```python
from build123d import *

# Parameters (mm, degrees)
ESQUISSE1_R             = 3
ESQUISSE1_R_2           = 2.5
BOSS_EXTRU_1_DEPTH      = 10
ESQUISSE4_W             = 8
ESQUISSE4_H             = 2
BOSS_EXTRU_2_DEPTH      = 8
CONG_1_R                = 3
ESQUISSE6_R             = 2
ENL_V_MAT_EXTRU_2_DEPTH = 12
BOSS_EXTRU_3_DEPTH      = 0.01
BOSS_EXTRU_3_DEPTH_BACK = 0.01
ESQUISSE7_R             = 2
ESQUISSE7_R_2           = 1.94261234


with BuildPart() as part:
    # Esquisse1 → Boss.-Extru.1 (new body)
    with BuildSketch(Plane.XY):
        Circle(ESQUISSE1_R)
        Circle(ESQUISSE1_R_2, mode=Mode.SUBTRACT)
    extrude(amount=BOSS_EXTRU_1_DEPTH)

    # Esquisse3 for Lissage3 → Lissage3 section 0
    with BuildSketch(Plane(origin=(0, 0, 0), x_dir=(-1, 0, 0), z_dir=(0, 0, -1))):
        with BuildLine():
            # circular arc as an exact rational Bezier (weights 1, cos(half-angle), 1)
            Bezier((-2.9104275, 0.727606875), (0, 12.369316884), (2.9104275, 0.727606875), weights=[1, 0.242535625, 1])
            Bezier((2.9104275, 0.727606875), (3.09232922, 0), (2.9104275, -0.727606875), weights=[1, 0.9701425, 1])
            Bezier((2.9104275, -0.727606875), (0, -12.369316884), (-2.9104275, -0.727606875), weights=[1, 0.242535625, 1])
            Bezier((-2.9104275, -0.727606875), (-3.09232922, 0), (-2.9104275, 0.727606875), weights=[1, 0.9701425, 1])
        make_face()
    # Esquisse2 → Lissage3 section 1
    with BuildSketch(Plane.XY.offset(-8)):
        with BuildLine():
            Line((4, 1), (-4, 1))
            Line((-4, 1), (-4, -1))
            Line((-4, -1), (4, -1))
            Line((4, -1), (4, 1))
        make_face()
    loft()

    # Esquisse4 → Boss.-Extru.2 (add)
    with BuildSketch(Plane(origin=(0, 0, -8), x_dir=(-1, 0, 0), z_dir=(0, 0, -1))):
        Rectangle(ESQUISSE4_W, ESQUISSE4_H)
    extrude(amount=BOSS_EXTRU_2_DEPTH)

    # Congé1
    cong_1_edges = [part.edges().sort_by_distance(p)[0] for p in [
        (-4, 0, -16),
        (4, 0, -16),
    ]]
    fillet(cong_1_edges, radius=CONG_1_R)

    # Esquisse6 → Enlèv. mat.-Extru.2 (cut)
    with BuildSketch(Plane(origin=(0, 1, 0), x_dir=(1, 0, 0), z_dir=(0, 1, 0))):
        with Locations(Location((0, 12, 0), (0, 0, 180))):
            Circle(ESQUISSE6_R)
    extrude(amount=-ENL_V_MAT_EXTRU_2_DEPTH, mode=Mode.SUBTRACT)

    # Esquisse7 → Boss.-Extru.3 (add, two sides: drawn at the far end of the back side and taken through both)
    with BuildSketch(Plane(origin=(0, 0, 0), x_dir=(1, 0, 0), z_dir=(0, 1, 0)).offset(-BOSS_EXTRU_3_DEPTH_BACK)):
        with Locations(Location((0, 12, 0), (0, 0, 180))):
            Circle(ESQUISSE7_R)
        with Locations(Location((0, 12, 0), (0, 0, 270))):
            Circle(ESQUISSE7_R_2, mode=Mode.SUBTRACT)
    extrude(amount=BOSS_EXTRU_3_DEPTH + BOSS_EXTRU_3_DEPTH_BACK)


solid = part.part
```
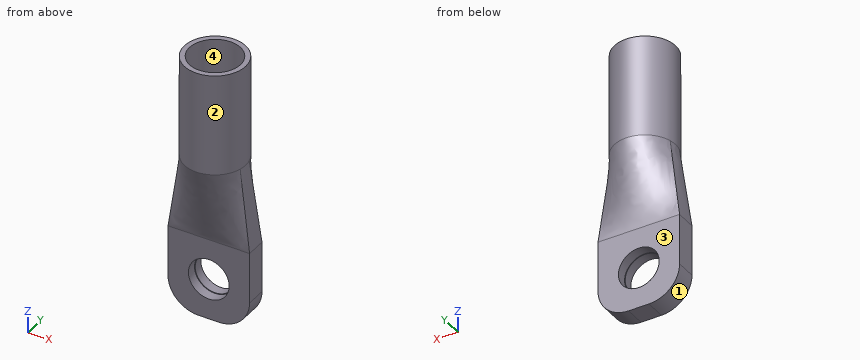
Here's how the part is built. I have some questions about the finished solid (model axes, mm). Face numbers are marked on the shaded views. Coordinates: 2 decimals unless noted, no trailing zeros. Order: outer loops, then holes, each group sorted by start corner. A loop starts at its lowest first (then second) coordinate and runs counter-clockwise, first axis right, second up.
Item 1: I need wall thicknesses on probe 1 along Z at (x, y) = (0, 0.85); probe 2 along Y at (x, z) = (-0.5, -8); probe 3 along X at (y, z) = (-1.25, 0.5). Which ranges of each line are inside material? Lowest first, please.
Response values:
probe 1: z = -16 to -14, -10 to 0
probe 2: y = -1 to 1
probe 3: x = -2.73 to -2.17, 2.17 to 2.73
Item 2: I'm going to push flat-ended pins straight in: pin 1 Ø1 at (y, z) = (2, 2) entering from +X; pin 2 Ø4.5 at (x, z) = (0, -12) entering from +Y; pin 3 Ø4 at (x, z) = (1, -12.5) entering from -Y; pin 4 Ø1 at (x, y) = (1.5, -0.5) entering from -Z. Where does each tip first touch, or does it pass through?
Response values:
pin 1: stops at x = 2.6
pin 2: stops at y = 1
pin 3: stops at y = -1
pin 4: stops at z = -16
Item 3: If we section it at B-B, the plane z = 3: List the corners of the cut face in (x, y) for me, then the cut area to 3 significant figures.
Response values:
outline: circle Ø6 at (0, 0); hole circle Ø5 at (0, 0)
area: 8.64 mm2
Item 4: Thinking about a two-plate mould opening in X: for the marked faces 1, 2, 3 and 4, which applies, pulls with the +X half, pulls with the -X half, needs draft (parallel to the pull), parting line crosses it, or undercut?
Response values:
face 1: pulls with the -X half
face 2: parting line crosses it
face 3: needs draft
face 4: undercut
